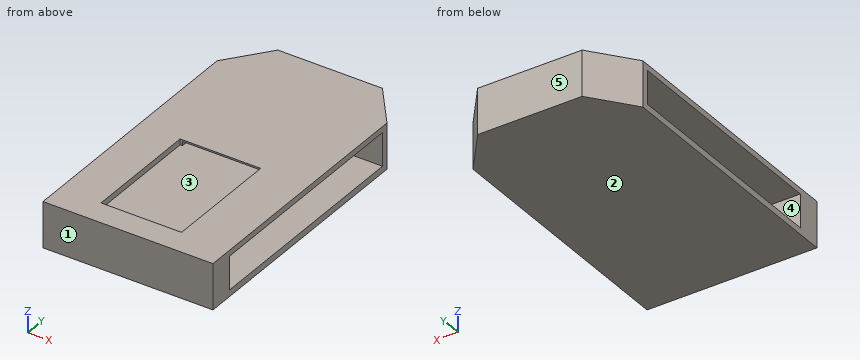
from build123d import *

# Parameters (mm, degrees)
BOSS_EXTRUDE1_DEPTH = 70
SKETCH2_W           = 123.25
SKETCH2_H           = 180
CUT_EXTRUDE1_DEPTH  = 60
SKETCH3_W           = 116.2609192
SKETCH3_H           = 54.96046542
CUT_EXTRUDE2_DEPTH  = 232
SKETCH4_W           = 51.18
SKETCH4_H           = 348.03
CUT_EXTRUDE3_DEPTH  = 260


with BuildPart() as part:
    # Sketch1 → Boss-Extrude1 (new body)
    with BuildSketch(Plane.XY):
        Polygon((130, -230), (-130, -230), (-130, 166.14), (-80, 230), (80, 230), (130, 166.14), align=None)
    extrude(amount=BOSS_EXTRUDE1_DEPTH)

    # Sketch2 → Cut-Extrude1 (cut)
    with BuildSketch(Plane.XY.offset(70)):
        with Locations((-5.475, -101.52)):
            Rectangle(SKETCH2_W, SKETCH2_H)
    extrude(amount=-CUT_EXTRUDE1_DEPTH, mode=Mode.SUBTRACT)

    # Sketch3 → Cut-Extrude2 (cut)
    with BuildSketch(Plane.XZ.offset(11.52)):
        with Locations((-5.475, 40)):
            Rectangle(SKETCH3_W, SKETCH3_H)
    extrude(amount=-CUT_EXTRUDE2_DEPTH, mode=Mode.SUBTRACT)

    # Sketch4 → Cut-Extrude3 (cut)
    with BuildSketch(Plane.ZY.offset(130)):
        with Locations((35.48, -18.055)):
            Rectangle(SKETCH4_W, SKETCH4_H)
    extrude(amount=-CUT_EXTRUDE3_DEPTH, mode=Mode.SUBTRACT)


solid = part.part
Build history of the part. All positions in model axes, mm. Face numbers are marked on the shaded views. A direction names the side the tool comes from. Round coordinates to 2 decimals unless told otherwise and drop trailing zeros. Write each loop counter-clockwise with the first axis right and the second up, starting at its lowest first coordinate (ties: lowest second). Pieces come first, ordered by that corner, then holes. Notation, with made-up numbers: M -9,26.25 L 46,26.25 A28 ccw 46,64.25 Z; hole C 51,6 d1. An arc over 180 degrees is marked long. Use CSV: the item, a comma, the result in double quotes.
1. Flat gauge pin, fed straight in: pin 1 (1.5 mm diameter, centred on y = -94.5, z = 59, fed in from +X). Where does the tip first touch, or does it go through?
Reply:
pin 1,"passes through"
2. Wall check: probe 1 along Y at (x, z) = (-15.5, 34); probe 2 along Y at (x, z) = (-79, 20.5); probe 3 along Z at (x, y) = (-36, -2). Give the ranges that are in metal, low to high. Write a range as from..to.
Reply:
probe 1,"y = -230..-192.07, 220.48..230"
probe 2,"y = -230..-192.07, 155.96..230"
probe 3,"z = 0..9.89, 67.48..70"
3. Two-plate mould, pull along Y, no slides. Class the marked faces 1, 2 and 3: +Y half, -Y half, draft (parallel to the pull), parting line (faces both ways), or undercut.
Reply:
face 1,"-Y half"
face 2,"draft"
face 3,"undercut"
4. Saw through at C-C (y = -73.5). Give the cut face in (x, z).
Reply:
outline,"M -130,0 L 130,0 L 130,9.89 L -130,9.89 Z; M -130,61.07 L -67.1,61.07 L -67.1,70 L -130,70 Z; M 56.15,61.07 L 130,61.07 L 130,70 L 56.15,70 Z"
5. Tool access for the marked faces 4 and 5: list every direction of +Z, -Z, +X, -X, +Y, -Y with a clear straight run to the whole face (end or side of a thin tool).
Reply:
face 4,"+X, -X"
face 5,"+Z, -Z, +X, -X, +Y"
6. Saw through at D-D (x = 63). Give the cut face in (y, z).
Reply:
outline,"M -230,0 L 230,0 L 230,70 L -230,70 Z; hole M -192.07,9.89 L 155.96,9.89 L 155.96,61.07 L -192.07,61.07 Z"
7. Saw through at B-B (z = 37.5). Give the cut face in (x, y), plus the area to 3 significant figures.
Reply:
outline,"M -130,-230 L 130,-230 L 130,-192.07 L -130,-192.07 Z; M -130,155.96 L -63.61,155.96 L -63.61,220.48 L 52.66,220.48 L 52.66,155.96 L 130,155.96 L 130,166.14 L 80,230 L -80,230 L -130,166.14 Z"
area,"18,400 mm²"
8. Saw through at A-A (y = 72). Give the cut face in (x, z).
Reply:
outline,"M -130,0 L 130,0 L 130,9.89 L -130,9.89 Z; M -130,61.07 L -63.61,61.07 L -63.61,67.48 L 52.66,67.48 L 52.66,61.07 L 130,61.07 L 130,70 L -130,70 Z"
